For this review, take the finished solid that the model builds, in its own axes (mm). Give positions to 0.01 mm unless a question says otherwise; leave off trailing zeros. Write each loop counter-clockwise with the first axis right and the second up, starting at its lowest first coordinate (ties: lowest second). Pieces come first, ordered by that corner, then holes. Notation, with made-up numbers: M 51.25,-36 L 64.25,-36 A19 ccw 64.25,-24 Z; hole C 89,29 d4. An arc over 180 degrees is marked long. Answer as a JSON object with one key per item and string values. Group by question number.
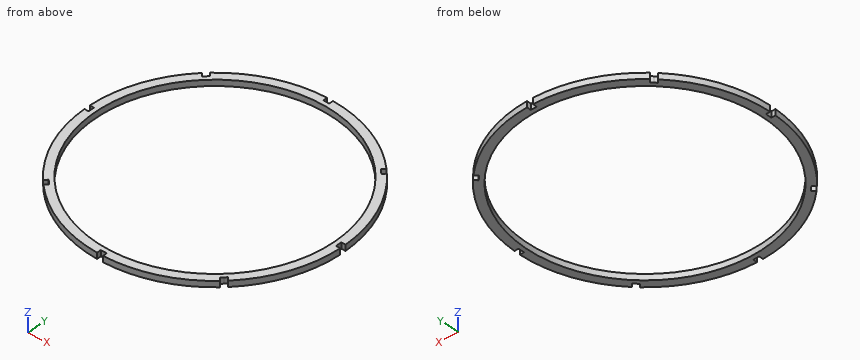
Autodesk Inventor part; units mm, degrees
ref_plane "YZ Plane" through (0, 0, 0) normal (1, 0, 0) x (0, 1, 0)
ref_plane "XZ Plane" through (0, 0, 0) normal (0, 1, 0) x (-1, 0, 0)
ref_plane "XY Plane" through (0, 0, 0) normal (0, 0, 1) x (1, 0, 0)
sketch "Sketch1" plane through (0, 0, 0) normal (0, 0, 1) x (1, 0, 0)
  circle A0 centre (0, 0) radius 70
  circle A1 centre (0, 0) radius 75
  line L0 (72.5, 1.75) -> (75, 1.75)
  line L1 (75, 1.75) -> (75, 0)
  line L2 (75, 0) -> (72.5, 0)
  line L3 (72.5, 0) -> (72.5, 1.75)
  line L4 (70, 0) -> (75, 0)
  line L5 (72.5, -1.75) -> (75, -1.75)
  line L6 (75, -1.75) -> (75, 0)
  line L7 (72.5, 0) -> (72.5, -1.75)
  line L8 (51.2652, 51.2652) -> (50.0278, 52.5027)
  line L9 (50.0278, 52.5027) -> (51.7956, 54.2704)
  line L10 (52.5027, 50.0278) -> (54.2704, 51.7956)
  line L11 (51.2652, 51.2652) -> (52.5027, 50.0278)
  line L12 (54.2704, 51.7956) -> (53.033, 53.033)
  line L13 (51.7956, 54.2704) -> (53.033, 53.033)
  line L14 (0, 72.5) -> (-1.75, 72.5)
  line L15 (-1.75, 72.5) -> (-1.75, 75)
  line L16 (1.75, 72.5) -> (1.75, 75)
  line L17 (0, 72.5) -> (1.75, 72.5)
  line L18 (1.75, 75) -> (0, 75)
  line L19 (-1.75, 75) -> (0, 75)
  line L20 (-51.2652, 51.2652) -> (-52.5027, 50.0278)
  line L21 (-52.5027, 50.0278) -> (-54.2704, 51.7956)
  line L22 (-50.0278, 52.5027) -> (-51.7956, 54.2704)
  line L23 (-51.2652, 51.2652) -> (-50.0278, 52.5027)
  line L24 (-51.7956, 54.2704) -> (-53.033, 53.033)
  line L25 (-54.2704, 51.7956) -> (-53.033, 53.033)
  line L26 (-72.5, 0) -> (-72.5, -1.75)
  line L27 (-72.5, -1.75) -> (-75, -1.75)
  line L28 (-72.5, 1.75) -> (-75, 1.75)
  line L29 (-72.5, 0) -> (-72.5, 1.75)
  line L30 (-75, 1.75) -> (-75, 0)
  line L31 (-75, -1.75) -> (-75, 0)
  line L32 (-51.2652, -51.2652) -> (-50.0278, -52.5027)
  line L33 (-50.0278, -52.5027) -> (-51.7956, -54.2704)
  line L34 (-52.5027, -50.0278) -> (-54.2704, -51.7956)
  line L35 (-51.2652, -51.2652) -> (-52.5027, -50.0278)
  line L36 (-54.2704, -51.7956) -> (-53.033, -53.033)
  line L37 (-51.7956, -54.2704) -> (-53.033, -53.033)
  line L38 (0, -72.5) -> (1.75, -72.5)
  line L39 (1.75, -72.5) -> (1.75, -75)
  line L40 (-1.75, -72.5) -> (-1.75, -75)
  line L41 (0, -72.5) -> (-1.75, -72.5)
  line L42 (-1.75, -75) -> (0, -75)
  line L43 (1.75, -75) -> (0, -75)
  line L44 (51.2652, -51.2652) -> (52.5027, -50.0278)
  line L45 (52.5027, -50.0278) -> (54.2704, -51.7956)
  line L46 (50.0278, -52.5027) -> (51.7956, -54.2704)
  line L47 (51.2652, -51.2652) -> (50.0278, -52.5027)
  line L48 (51.7956, -54.2704) -> (53.033, -53.033)
  line L49 (54.2704, -51.7956) -> (53.033, -53.033)
  point P0 (74.9796, 1.75)
  point P1 (54.256, 51.7811)
  point P2 (51.7811, 54.256)
  point P3 (1.75, 74.9796)
  point P4 (-1.75, 74.9796)
  point P5 (-51.7811, 54.256)
  point P6 (-54.256, 51.7811)
  point P7 (-74.9796, 1.75)
  point P8 (-74.9796, -1.75)
  point P9 (-54.256, -51.7811)
  point P10 (-51.7811, -54.256)
  point P11 (-1.75, -74.9796)
  point P12 (1.75, -74.9796)
  point P13 (51.7811, -54.256)
  point P14 (54.256, -51.7811)
  point P15 (74.9796, -1.75)
  dimension "d0" = 140
  dimension "d1" = 5
  dimension "d2" = 1.75
  dimension "d5" = 360
extrude "Extrusion1" add sketch "Sketch1" along normal mid plane 3.5 contours L7 L5 A1 L45 L44 L47 L46 L39 L38 L41 L40 L33 L32 L35 L34 L27 L26 L29 L28 L21 L20 L23 L22 L15 L14 L17 L16 L9 L8 L11 L10 L0 L3
properties part number "Sirsi obroc"
Item 1: Consider section A-A (x = 0). Give the boundary of the cut face in (y, z), plus the area to 3 significant figures.
Item 2: To check wall thickness, follow probe 1 along Y at (x, z) = (0, 0.15); probe 2 along Y at (x, z) = (-29.5, 1.5); probe 3 along X at (y, z) = (-22, 0.1). State the ranges of each line that lie inside material, in increasing order.
Item 3: Insertion check: P1, Ø1.8, axis at y = 0, z = 0.5, coming from the +X side; P2, Ø1, axis at x = 0.5, z = 0.5, coming from the +Y side; P3, Ø1, axis at x = 27.5, z = -0.5, coming from the +Y side. Each pin has a flat end and moves straight along its axis. Give the tip position at first contact, or say it passes through.
Result set:
{
 "1": {"outline": "M -72.5,-1.75 L -70,-1.75 L -70,1.75 L -72.5,1.75 Z; M 70,-1.75 L 72.5,-1.75 L 72.5,1.75 L 70,1.75 Z", "area": "17.5 mm^2"},
 "2": {"probe 1": "y = -72.5 to -70, 70 to 72.5", "probe 2": "y = -68.95 to -63.48, 63.48 to 68.95", "probe 3": "x = -71.7 to -66.45, 66.45 to 71.7"},
 "3": {"P1": "stops at x = 72.5", "P2": "stops at y = 72.5", "P3": "stops at y = 69.97"}
}
